Check sheet for the modelled part. Datum: model origin and axes. Units: mm. Round coordinates to 2 decimals unless told otherwise and drop trailing zeros. Order: outer loops, then holes, each group sorted by start corner. A loop starts at its lowest first (then second) coordinate and runs counter-clockwise, first axis right, second up. Notation, with made-up numbers: (27, 66) -> (85, 66) arc R32 cw to (85, 92) -> close; hole circle Ø1 at (78.25, 78). An arc over 180 degrees is marked (long way). Answer in a Markdown table with one row per item.
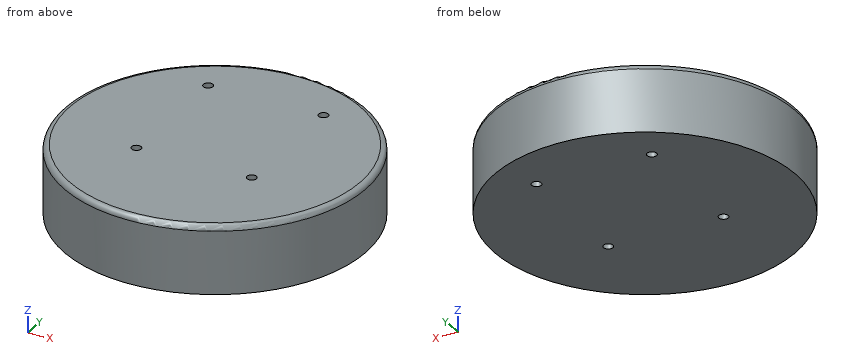
```python
from build123d import *

# Parameters (mm, degrees)
F0_R     = 55
F1_DEPTH = 25
F2_R     = 2
F3_R     = 1.75
F4_DEPTH = 25


with BuildPart() as f1:
    # F0 (on Top) → F1 (new body)
    with BuildSketch(Plane.XY):
        Circle(F0_R)
    extrude(amount=F1_DEPTH)

    # F2
    f2_edges = [f1.edges().sort_by_distance(p)[0] for p in [
        (-55, 0, 25),
    ]]
    fillet(f2_edges, radius=F2_R)

    # F3 (on face) → F4 (cut, through all)
    with BuildSketch(Plane.XY.offset(25)):
        with Locations((-21, 34)):
            Circle(F3_R)
        with Locations((21, 34)):
            Circle(F3_R)
        with Locations((21, -14)):
            Circle(F3_R)
        with Locations((-21, -14)):
            Circle(F3_R)
    extrude(amount=-F4_DEPTH, mode=Mode.SUBTRACT)


solid = f1.part
```
(1) Scan lines: probe 1 along Y at (x, z) = (-21, 7.5); probe 2 along X at (y, z) = (-13.5, 6); probe 3 along X at (y, z) = (-13, 11.25). Record each from-to range of solid material in increasing order. Write a range as from..to.
Solutions:
| item | result |
|---|---|
| probe 1 | -50.83..-15.75, -12.25..32.25, 35.75..50.83 |
| probe 2 | -53.32..-22.68, -19.32..19.32, 22.68..53.32 |
| probe 3 | -53.44..-22.44, -19.56..19.56, 22.44..53.44 |
(2) Section check A-A on z = 5. Record the boundary of the cut face in (x, y), plus the area to 3 significant figures.
Solutions:
| item | result |
|---|---|
| outline | circle Ø110 at (0, 0); hole circle Ø3.5 at (-21, -14); hole circle Ø3.5 at (-21, 34); hole circle Ø3.5 at (21, -14); hole circle Ø3.5 at (21, 34) |
| area | 9,460 mm^2 |
(3) Depth check by flat-ended pin: pin 1 Ø3 at (x, z) = (13.5, 5) entering from +Y; pin 2 Ø2 at (y, z) = (3, 18) entering from -X; pin 3 Ø8 at (y, z) = (-6.5, 3.5) entering from +X. Enter the tip coordinate at first touch or a pass-through.
Solutions:
| item | result |
|---|---|
| pin 1 | y = 53.67 |
| pin 2 | x = -54.96 |
| pin 3 | x = 54.94 |
(4) Section check B-B on x = -21. Give the number of separate pieces and of enclosed holes in the cut face, plus the area to 3 significant figures.
Solutions:
| item | result |
|---|---|
| separate pieces | 3 |
| enclosed holes | 0 |
| area | 2,360 mm^2 |
